Design review of the part built by this model. Coordinates are the model's own, in mm. A direction names the side the tool comes from. Give positions to 0.01 mm unless a question says otherwise; leave off trailing zeros. Write each loop counter-clockwise with the first axis right and the second up, starting at its lowest first coordinate (ties: lowest second). Pieces come first, ordered by that corner, then holes.
```python
from build123d import *

# Parameters (mm, degrees)
EXTRUDE_1_DEPTH     = 2
SKETCH_2_R          = 1.1
EXTRUDE_2_DEPTH     = 3
SKETCH_3_R          = 3.75
EXTRUDE_3_DEPTH     = 5
CHAMFER_1_SIZE      = 0.8
SKETCH_4_R          = 1.1
CUT_EXTRUDE_1_DEPTH = 4
SKETCH_5_R          = 2.25
CUT_EXTRUDE_2_DEPTH = 1.5


with BuildPart() as part:
    # 草图1 → 凸台-拉伸1 (new body)
    with BuildSketch(Plane.XY):
        with BuildLine():
            Line((-2.189141888, -0.35), (-2.65, -6.47746827))
            Line((-2.65, -6.47746827), (2.65, -6.47746827))
            Line((2.65, -6.47746827), (2.189141888, -0.35))
            ThreePointArc((2.189141888, -0.35), (1.554921872, 0.96628783), (0.194774821, 1.5))
            Line((0.194774821, 1.5), (-0.194774821, 1.5))
            ThreePointArc((-0.194774821, 1.5), (-1.554921872, 0.96628783), (-2.189141888, -0.35))
        make_face()
    extrude(amount=EXTRUDE_1_DEPTH)

    # 草图2 → 凸台-拉伸2 (add)
    with BuildSketch(Plane.XY.offset(2)):
        with Locations(Location((0, 0, 0), (0, 0, 180))):
            Circle(SKETCH_2_R)
    extrude(amount=EXTRUDE_2_DEPTH)

    # 草图3 → 凸台-拉伸3 (add)
    with BuildSketch(Plane.XY):
        with Locations(Location((0, -7, 0), (0, 0, 131.352385807))):
            Circle(SKETCH_3_R)
    extrude(amount=EXTRUDE_3_DEPTH)

    # 倒角1
    chamfer_1_edges = [part.edges().sort_by_distance(p)[0] for p in [
        (2.477581037, -9.814976413, 5),
    ]]
    chamfer(chamfer_1_edges, length=CHAMFER_1_SIZE)

    # 草图4 → 切除-拉伸1 (cut)
    with BuildSketch(Plane(origin=(0, 0, 0), x_dir=(-1, 0, 0), z_dir=(0, 0, -1))):
        with Locations((0, -7)):
            Circle(SKETCH_4_R)
    extrude(amount=-CUT_EXTRUDE_1_DEPTH, mode=Mode.SUBTRACT)

    # 草图5 → 切除-拉伸2 (cut)
    with BuildSketch(Plane(origin=(0, 0, 0), x_dir=(-1, 0, 0), z_dir=(0, 0, -1))):
        with Locations((0, -7)):
            Circle(SKETCH_5_R)
    extrude(amount=-CUT_EXTRUDE_2_DEPTH, mode=Mode.SUBTRACT)


solid = part.part
```
(1) Tool access review of faces 4 (the face through (1, -4, 0)), 5 (the face through (0, -7, 4)), 6 (the face through (-0.08, -10.75, 2.07)): name each direction out of +Z, -Z, +X, -X, +Y, -Y from which nothing blocks a thin tool from reaching the whole face with its end or side.
Resolved:
face 4: -Z, +X, -X, +Y, -Y
face 5: -Z
face 6: +Z
(2) Clearance check with flat-ended pins moving along their axes: P1, Ø2, axis at x = -1, y = -7, coming from the -Z side; P2, Ø1.5, axis at x = 2, z = 3, coming from the -Y side; P3, Ø0.7, axis at x = -0.5, y = -6.5, coming from the -Z side. State where each tip first meets the part, or that it passes through.
Resolved:
P1: stops at z = 1.5
P2: stops at y = -10.54
P3: stops at z = 4
(3) Consider section A-A, the plane z = 1.3. Give the boundary of the cut face in (x, y), then the cut area to 3 significant figures.
Resolved:
outline: (-2.48, -4.19) arc R3.75 ccw (long way) to (2.48, -4.19) - (2.19, -0.35) arc R2 ccw to (0.19, 1.5) - (-0.19, 1.5) arc R2 ccw to (-2.19, -0.35) - close; hole circle Ø4.5 at (0, -7)
area: 49.4 mm2
(4) Consider section B-B, the plane z = 2.2. Give the boundary of the cut face in (x, y), then the cut area to 3 significant figures.
Resolved:
outline: circle Ø7.5 at (0, -7); circle Ø2.2 at (0, 0); hole circle Ø2.2 at (0, -7)
area: 44.2 mm2
(5) Consider section D-D, the plane x = 0. Give the boundary of the cut face in (y, z).
Resolved:
outline: (-10.75, 0) - (-9.25, 0) - (-9.25, 1.5) - (-8.1, 1.5) - (-8.1, 4) - (-5.9, 4) - (-5.9, 1.5) - (-4.75, 1.5) - (-4.75, 0) - (1.5, 0) - (1.5, 2) - (1.1, 2) - (1.1, 5) - (-1.1, 5) - (-1.1, 2) - (-3.25, 2) - (-3.25, 4.2) - (-4.05, 5) - (-9.95, 5) - (-10.75, 4.2) - close
(6) Consider section C-C, the plane y = -7. Give the boundary of the cut face in (x, z), then the cut area to 3 significant figures.
Resolved:
outline: (-3.75, 0) - (-2.25, 0) - (-2.25, 1.5) - (-1.1, 1.5) - (-1.1, 4) - (1.1, 4) - (1.1, 1.5) - (2.25, 1.5) - (2.25, 0) - (3.75, 0) - (3.75, 4.2) - (2.95, 5) - (-2.95, 5) - (-3.75, 4.2) - close
area: 24.6 mm2
(7) Mouldability with a two-part tool opening along Y and no side actions: class faces 1 (the face through (0, 0, 5)), 2 (the face through (0.238, -8.074, 2.732)), 3 (the face through (2.335, -2.294, 0.986)) as pulls with the +Y half, pulls with the -Y half, needs draft (parallel to the pull), parting line crosses it, or undercut.
Resolved:
face 1: needs draft
face 2: undercut
face 3: pulls with the +Y half
(8) To check wall thickness, follow L1, parallel to Y at x = 0, z = 3.45; L2, parallel to Y at x = 0, z = 1; L3, parallel to Z at x = 1, y = 0.75. State the ranges of each line that lie inside material, in increasing order.
Resolved:
L1: y = -10.75 to -8.1, -5.9 to -3.25, -1.1 to 1.1
L2: y = -10.75 to -9.25, -4.75 to 1.5
L3: z = 0 to 2
